Verification items for the finished model (mm, model axes). A direction names the side the tool comes from. Round coordinates to 2 decimals unless told otherwise and drop trailing zeros. Loops run counter-clockwise (first coordinate to the right, second up) from the corner with the lowest first, then second, coordinate; pieces in that order, holes last.
from build123d import *

# Parameters (mm, degrees)
BOSS_EXTRUDE1_DEPTH  = 2
BOSS_EXTRUDE6_DEPTH  = 4.5
CUT_EXTRUDE6_DEPTH   = 4.5
BOSS_EXTRUDE14_DEPTH = 2.3
SKETCH32_R           = 3
CUT_EXTRUDE7_DEPTH   = 2.3
SKETCH33_W           = 17.343145750507624
SKETCH33_H           = 2
BOSS_EXTRUDE15_DEPTH = 1.2
CUT_EXTRUDE8_DEPTH   = 2.4
CUT_EXTRUDE9_DEPTH   = 4.3999999999999995
SKETCH37_R           = 3.899999999999994
BOSS_EXTRUDE16_DEPTH = 4.4
CUT_EXTRUDE10_DEPTH  = 39.60291748102272
SKETCH43_R           = 2.5000000000000004
SKETCH43_R_2         = 2.4999999999999982
BOSS_EXTRUDE17_DEPTH = 1.2
SKETCH44_R           = 0.9499999999999992
SKETCH44_R_2         = 0.9500000000000008
CUT_EXTRUDE11_DEPTH  = 40.360198653546576
SKETCH45_R           = 1.9999999999999996
SKETCH45_R_2         = 2.000000000000003
CUT_EXTRUDE12_DEPTH  = 4.5
SKETCH49_R           = 0.7500000000000021
CUT_EXTRUDE13_DEPTH  = 3
CUT_EXTRUDE14_DEPTH  = 6.8
FILLET1_R            = 1.5
FILLET3_R            = 1


with BuildPart() as part:
    # Sketch3 → Boss-Extrude1 (new body)
    with BuildSketch(Plane.XY):
        with BuildLine():
            Line((8.000000000000002, 0), (8.999999999999993, -2.5431457505076343))
            Line((8.999999999999993, -2.5431457505076343), (8.999999999999993, -7.04314575050762))
            Line((8.999999999999993, -7.04314575050762), (21.50000000000003, -7.043145750507617))
            Line((21.50000000000003, -7.043145750507617), (25.05025253169419, -4.949747468305846))
            ThreePointArc((25.05025253169419, -4.949747468305846), (36.46715672757901, -2.678784026555599), (30, 7.000000000000014))
            Line((30, 7.000000000000014), (26.999999999999996, 7.456854249492377))
            Line((26.999999999999996, 7.456854249492377), (5.656854249492369, 7.456854249492377))
            Line((5.656854249492369, 7.456854249492377), (5.656854249492376, 5.656854249492382))
            ThreePointArc((5.656854249492376, 5.656854249492382), (7.391036260090296, 3.061467458920721), (8.000000000000002, 0))
        make_face()
    extrude(amount=BOSS_EXTRUDE1_DEPTH)

    # Sketch22 → Boss-Extrude6 (add)
    with BuildSketch(Plane.XY.offset(2)):
        with BuildLine():
            Line((5.656854249492376, 7.456854249492377), (21.50000000000004, 7.456854249492377))
            Line((21.50000000000004, 7.456854249492377), (26.999999999999996, 7.456854249492377))
            Line((26.999999999999996, 7.456854249492377), (26.999999999999996, 2.1288604946885763))
            Line((26.999999999999996, 2.1288604946885763), (23.27512626584711, 2.128860494688576))
            Line((23.27512626584711, 2.128860494688576), (23.27512626584711, -5.996446609406731))
            Line((23.27512626584711, -5.996446609406731), (21.50000000000003, -7.043145750507617))
            Line((21.50000000000003, -7.043145750507617), (8.999999999999993, -7.04314575050762))
            Line((8.999999999999993, -7.04314575050762), (8.999999999999993, -2.5431457505076343))
            Line((8.999999999999993, -2.5431457505076343), (7.999999999999998, 0))
            ThreePointArc((7.999999999999998, 0), (7.391036260090291, 3.061467458920719), (5.656854249492376, 5.656854249492382))
            Line((5.656854249492376, 5.656854249492382), (5.656854249492376, 7.456854249492377))
        make_face()
    extrude(amount=BOSS_EXTRUDE6_DEPTH)

    # Sketch26 → Cut-Extrude6 (cut)
    with BuildSketch(Plane.XY.offset(2)):
        Polygon((18.098080447707712, 5.299999999999999), (2.5300524575164793, 5.299999999999999), (2.5300524575164793, 4), (18.098080447707712, 4), (26.999999999999996, 4), (26.999999999999996, 5.299999999999999), align=None)
    extrude(amount=CUT_EXTRUDE6_DEPTH, mode=Mode.SUBTRACT)


with BuildPart() as body_2:
    # Sketch31 → Boss-Extrude14 (new body)
    with BuildSketch(Plane.XY.offset(6.5)):
        with BuildLine():
            Line((2.4326880657739025, 5.656854249492382), (0, 5.656854249492382))
            ThreePointArc((0, 5.656854249492382), (-5.656854249492382, 6.9e-16), (0, -5.656854249492382))
            Line((0, -5.656854249492382), (9.000000000000004, -5.656854249492382))
            Line((9.000000000000004, -5.656854249492382), (8.999999999999993, -7.04314575050762))
            Line((8.999999999999993, -7.04314575050762), (8.999999999999993, -8.54314575050762))
            Line((8.999999999999993, -8.54314575050762), (21.50000000000003, -8.54314575050762))
            Line((21.50000000000003, -8.54314575050762), (21.50000000000003, -7.043145750507617))
            Line((21.50000000000003, -7.043145750507617), (23.27512626584711, -5.996446609406731))
            Line((23.27512626584711, -5.996446609406731), (23.27512626584711, 2.128860494688576))
            Line((23.27512626584711, 2.128860494688576), (26.999999999999996, 2.1288604946885763))
            Line((26.999999999999996, 2.1288604946885763), (26.999999999999996, 7.456854249492377))
            Line((26.999999999999996, 7.456854249492377), (26.999999999999996, 8.956854249492377))
            Line((26.999999999999996, 8.956854249492377), (5.656854249492376, 8.956854249492377))
            Line((5.656854249492376, 8.956854249492377), (5.656854249492376, 7.456854249492377))
            Line((5.656854249492376, 7.456854249492377), (5.656854249492376, 5.656854249492382))
            Line((5.656854249492376, 5.656854249492382), (2.4326880657739025, 5.656854249492382))
        make_face()
    extrude(amount=BOSS_EXTRUDE14_DEPTH)

    # Sketch32 → Cut-Extrude7 (cut)
    with BuildSketch(Plane.XY.offset(8.799999999999999)):
        Circle(SKETCH32_R)
    extrude(amount=-CUT_EXTRUDE7_DEPTH, mode=Mode.SUBTRACT)

    # Sketch33 → Boss-Extrude15 (add)
    with BuildSketch(Plane.XY.offset(8.799999999999999)):
        with Locations((14.328427124746185, 7.956854249492377)):
            Rectangle(SKETCH33_W, SKETCH33_H)
        Polygon((9.000000000000004, -7.043145750507619), (9.000000000000004, -8.54314575050762), (21.50000000000003, -8.54314575050762), (21.50000000000003, -7.043145750507617), align=None)
        with BuildLine():
            Line((7.000000000000003, -4.156854249492383), (23.275126265847117, -4.156854249492383))
            Line((23.275126265847117, -4.156854249492383), (23.275126265847113, -2.1568542494923815))
            Line((23.275126265847113, -2.1568542494923815), (7.000000000000003, -2.1568542494923832))
            ThreePointArc((7.000000000000003, -2.1568542494923832), (6.000000000000003, -3.1568542494923832), (7.000000000000003, -4.156854249492383))
        make_face()
        with BuildLine():
            Line((18.999999999999996, 2.172006245196199), (7.000000000000003, 2.172006245196201))
            ThreePointArc((7.000000000000003, 2.172006245196201), (6.0000000000000036, 3.1720062451962), (7.000000000000003, 4.172006245196199))
            Line((7.000000000000003, 4.172006245196199), (18.999999999999996, 4.172006245196199))
            Line((18.999999999999996, 4.172006245196199), (18.999999999999996, 2.172006245196199))
        make_face()
    extrude(amount=BOSS_EXTRUDE15_DEPTH)


with BuildPart() as cut_extrude8_tool:
    # Sketch35 → Cut-Extrude8 (new body)
    with BuildSketch(Plane.XY.offset(8.799999999999999)):
        Polygon((26.999999999999996, 2.1288604946885763), (26.999999999999996, 6.000000000000002), (21.520354003499165, 6.000000000000002), (21.520354003499165, 2.1288604946885754), align=None)
    extrude(amount=-CUT_EXTRUDE8_DEPTH)


with BuildPart() as part_1:
    add(part.part)

    # Cut-Extrude8: cut by cut_extrude8_tool
    add(cut_extrude8_tool.part, mode=Mode.SUBTRACT)

    # Sketch36 → Cut-Extrude9 (cut)
    with BuildSketch(Plane.XY.offset(6.3999999999999995)):
        Polygon((26.999999999999996, 2.1288604946885763), (26.999999999999996, 4), (23.30000000000004, 3.999999999999999), (23.30000000000003, 2.1288604946885754), align=None)
    extrude(amount=-CUT_EXTRUDE9_DEPTH, mode=Mode.SUBTRACT)

    # Sketch37 → Boss-Extrude16 (add)
    with BuildSketch(Plane.XY.offset(2)):
        with Locations((29.999999999999996, 1.388e-14)):
            Circle(SKETCH37_R)
    extrude(amount=BOSS_EXTRUDE16_DEPTH)

    # Sketch39 → Cut-Extrude10 (cut, through all)
    with BuildSketch(Plane.XY.offset(6.4)):
        with BuildLine():
            Line((28.999999999999993, 0.9797958971132569), (28.999999999999993, -0.9797958971132569))
            ThreePointArc((28.999999999999993, -0.9797958971132569), (31.4, 2.383e-14), (28.999999999999993, 0.9797958971132569))
        make_face()
    extrude(amount=-CUT_EXTRUDE10_DEPTH, mode=Mode.SUBTRACT)


with BuildPart() as body_2_1:
    add(body_2.part)

    # Cut-Extrude8: cut by cut_extrude8_tool
    add(cut_extrude8_tool.part, mode=Mode.SUBTRACT)

    # Sketch43 → Boss-Extrude17 (add)
    with BuildSketch(Plane.XY.offset(8.799999999999999)):
        with Locations((11.500000000000004, 0)):
            Circle(SKETCH43_R)
        with Locations((18.000000000000004, 0)):
            Circle(SKETCH43_R_2)
    extrude(amount=BOSS_EXTRUDE17_DEPTH)


with BuildPart() as cut_extrude11_tool:
    # Sketch44 → Cut-Extrude11 (new, through all)
    with BuildSketch(Plane.XY.offset(9.999999999999998)):
        with Locations((11.500000000000004, 0)):
            Circle(SKETCH44_R)
        with Locations((18.000000000000004, 0)):
            Circle(SKETCH44_R_2)
    extrude(amount=-CUT_EXTRUDE11_DEPTH)


with BuildPart() as part_2:
    add(part_1.part)

    # Cut-Extrude11: cut by cut_extrude11_tool
    add(cut_extrude11_tool.part, mode=Mode.SUBTRACT)

    # Sketch45 → Cut-Extrude12 (cut)
    with BuildSketch(Plane(origin=(0, 0, 0), x_dir=(-1, 0, 0), z_dir=(0, 0, -1))):
        with Locations((-11.500000000000004, 0)):
            Circle(SKETCH45_R)
        with Locations((-18.000000000000004, 0)):
            Circle(SKETCH45_R_2)
    extrude(amount=-CUT_EXTRUDE12_DEPTH, mode=Mode.SUBTRACT)


with BuildPart() as body_2_2:
    add(body_2_1.part)

    # Cut-Extrude11: cut by cut_extrude11_tool
    add(cut_extrude11_tool.part, mode=Mode.SUBTRACT)

    # Sketch49 → Cut-Extrude13 (cut)
    with BuildSketch(Plane.XZ.offset(-6.956854249492377)):
        with Locations((19.999999999999996, 9.999999999999998)):
            Circle(SKETCH49_R)
    extrude(amount=-CUT_EXTRUDE13_DEPTH, mode=Mode.SUBTRACT)


with BuildPart() as cut_extrude14_tool:
    # Sketch51 → Cut-Extrude14 (new body)
    with BuildSketch(Plane.XY.offset(8.799999999999999)):
        Polygon((27, 8.956854249492377), (24.058650564533934, 8.956854249492377), (24.058650564533938, 4.991269007681976), (26.999999999999996, 4.991269007681976), align=None)
    extrude(amount=-CUT_EXTRUDE14_DEPTH)


with BuildPart() as part_3:
    add(part_2.part)

    # Cut-Extrude14: cut by cut_extrude14_tool
    add(cut_extrude14_tool.part, mode=Mode.SUBTRACT)

    # Fillet3
    fillet3_edges = [part_3.edges().sort_by_distance(p)[0] for p in [
        (23.27512626584711, -5.996446609406731, 4.25),
        (24.058650564533934, 7.456854249492377, 4.25),
        (8.999999999999993, -7.04314575050762, 3.25),
        (5.656854249492373, 7.456854249492377, 3.25),
        (15.25000000000001, -7.043145750507618, 0),
        (16.328427124746185, 7.456854249492377, 0),
    ]]
    fillet(fillet3_edges, radius=FILLET3_R)


with BuildPart() as body_2_3:
    add(body_2_2.part)

    # Cut-Extrude14: cut by cut_extrude14_tool
    add(cut_extrude14_tool.part, mode=Mode.SUBTRACT)

    # Fillet1
    fillet1_edges = [body_2_3.edges().sort_by_distance(p)[0] for p in [
        (14.857752407013155, 8.956854249492377, 6.5),
        (15.25000000000001, -8.54314575050762, 6.5),
    ]]
    fillet(fillet1_edges, radius=FILLET1_R)


solid = body_2_3.part
1. Gauge pin test, flat ends, axial feed: P1, Ø3, axis at x = 3.5, y = -1.5, coming from the +Z side; P2, Ø1.8, axis at x = 4, z = 8, coming from the -Y side; P3, Ø0.8, axis at y = -8, z = 8, coming from the +X side; P4, Ø8, axis at x = 4.5, y = 3.5, coming from the +Z side. Record the tip position at first contact, or that the pin passes through.
2. Section check C-C (x = 16). Enter the section's corners in (y, z).
3. Tool access check on faces 5 (the face through (19.98, 7.94, 9.25)), 6 (the face through (6, 3.2, 9.4)), 7 (the face through (5.657, 7, 8)), 8 (the face through (22, 2.129, 8)). Record the directions out of +Z, -Z, +X, -X, +Y, -Y that give a thin tool (end or side, any length) a straight path to the whole face; none if there is none.
4. Scan lines: L1, parallel to Y at x = 11.5, z = 9.2; L2, parallel to Y at x = 11.5, z = 8.2; L3, parallel to Y at x = 0, z = 7.7. Record each from-to range of solid material in increasing order.
5. Section check B-B (x = 11.5). Enter the section's corners in (y, z).
6. Section check D-D (z = 7.5). Enter the section's corners in (x, y), then the cut area to 3 significant figures.
7. Release check for a two-part mould opening along Y. For faces 1 (the face through (14, 0, 9)), 2 (the face through (-5.655, 0.124, 7.634)), 3 (the face through (3, 5.657, 8)), 4 (the face through (9, -7, 8)) record: released by +Y, released by -Y, zero draft, split by the parting line, or undercut.
8. Section check A-A (y = 0). Enter the section's corners in (x, z), then the cut area to 3 significant figures.
Taken from the geometry:
1. P1: stops at z = 8.8
1. P2: stops at y = -5.66
1. P3: stops at x = 21.5
1. P4: stops at z = 10
2. outline: (-8.54, 8) arc R1.5 ccw to (-7.04, 6.5) - (7.46, 6.5) arc R1.5 ccw to (8.96, 8) - (8.96, 10) - (6.96, 10) - (6.96, 8.8) - (4.17, 8.8) - (4.17, 10) - (2.17, 10) - (2.17, 8.8) - (1.5, 8.8) - (1.5, 10) - (-1.5, 10) - (-1.5, 8.8) - (-2.16, 8.8) - (-2.16, 10) - (-4.16, 10) - (-4.16, 8.8) - (-7.04, 8.8) - (-7.04, 10) - (-8.54, 10) - close
3. face 5: +Z, +Y
3. face 6: +Z, -X
3. face 7: +Z, -Z, -X, +Y
3. face 8: +Z, -Z, +X
4. L1: y = -8.54 to -7.04, -4.16 to -0.95, 0.95 to 4.17, 6.96 to 8.96
4. L2: y = -8.54 to -0.95, 0.95 to 8.96
4. L3: y = -5.66 to -3, 3 to 5.66
5. outline: (-8.54, 8) arc R1.5 ccw to (-7.04, 6.5) - (-0.95, 6.5) - (-0.95, 10) - (-4.16, 10) - (-4.16, 8.8) - (-7.04, 8.8) - (-7.04, 10) - (-8.54, 10) - close; (0.95, 6.5) - (7.46, 6.5) arc R1.5 ccw to (8.96, 8) - (8.96, 10) - (6.96, 10) - (6.96, 8.8) - (4.17, 8.8) - (4.17, 10) - (0.95, 10) - close
6. outline: (0, -5.66) - (9, -5.66) - (9, -8.46) - (21.5, -8.46) - (21.5, -7.04) - (23.28, -6) - (23.28, 2.13) - (21.52, 2.13) - (21.52, 6) - (24.06, 6) - (24.06, 8.87) - (5.66, 8.87) - (5.66, 5.66) - (0, 5.66) arc R5.66 ccw to start; hole circle Ø6 at (0, 0); hole circle Ø1.9 at (11.5, 0); hole circle Ø1.9 at (18, 0)
6. area: 368 mm2
7. face 1: undercut
7. face 2: split by the parting line
7. face 3: released by +Y
7. face 4: zero draft
8. outline: (-5.66, 6.5) - (-3, 6.5) - (-3, 8.8) - (-5.66, 8.8) - close; (3, 6.5) - (10.55, 6.5) - (10.55, 10) - (9, 10) - (9, 8.8) - (3, 8.8) - close; (12.45, 6.5) - (17.05, 6.5) - (17.05, 10) - (15.5, 10) - (15.5, 8.8) - (14, 8.8) - (14, 10) - (12.45, 10) - close; (18.95, 6.5) - (23.28, 6.5) - (23.28, 8.8) - (20.5, 8.8) - (20.5, 10) - (18.95, 10) - close
8. area: 51.4 mm2
